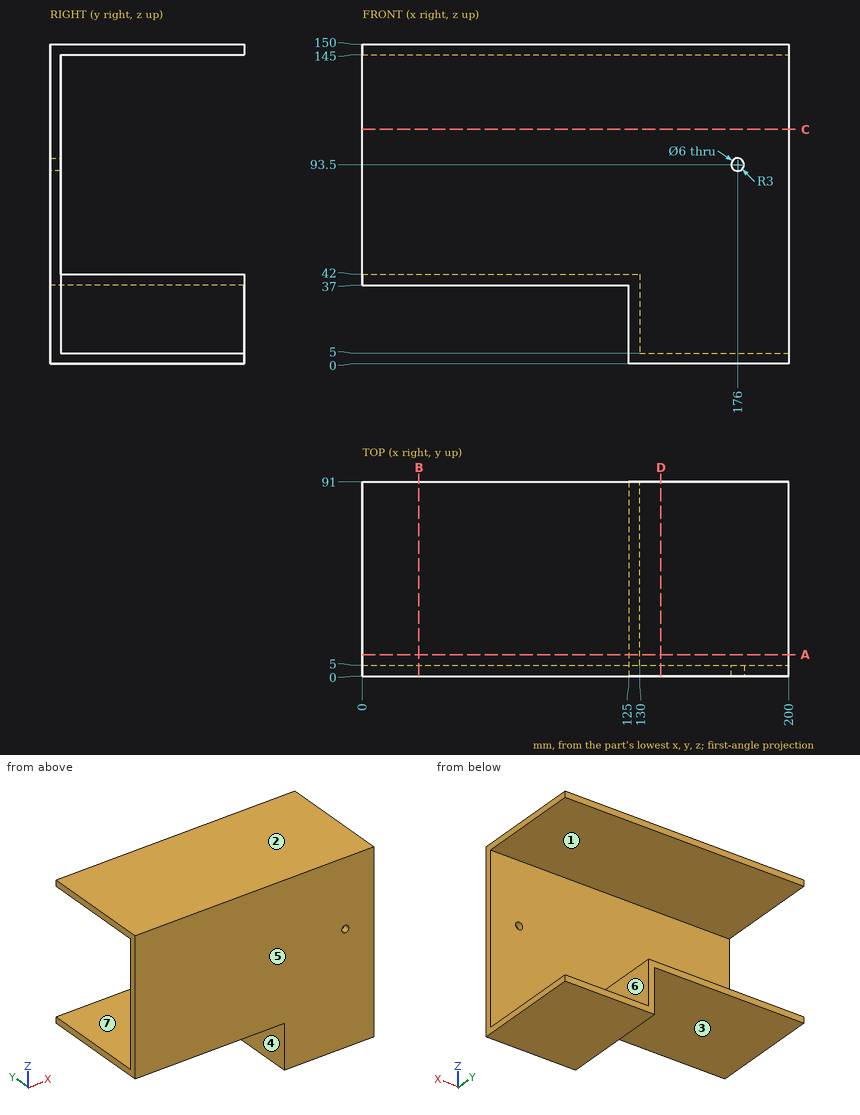
The drawing under review shows one solid part. Ordinate dimensions are in mm from its lowest x, y, z. A direction names the side the tool comes from. Round coordinates to 2 decimals unless told otherwise and drop trailing zeros. Loops run counter-clockwise (first coordinate to the right, second up) from the corner with the lowest first, then second, coordinate; pieces in that order, holes last. Notation, with made-up numbers: (9.5, -12.5) - (39.5, -12.5) arc R21 ccw to (39.5, 6.5) - close; hole circle Ø11 at (63, 5.5). An arc over 180 degrees is marked (long way). Use a Markdown table: item, result. Add a question column.
Q1. Add section B-B (x = 26.5). State the section outline as (y, z) points.
Q2. Add section D-D (x = 140). State the section outline as (y, z) points.
Q3. The part is to be moulded in two halves that separate along Z. For the marked faces 1, 2, 3 and 4, say which applies: pulls with the +Z half, pulls with the -Z half, needs draft (parallel to the pull), parting line crosses it, or undercut.
Q4. Add section C-C (z = 110). State the section outline as (x, y) points, plus the area to 3 significant figures.
Q5. Insertion check: pin 1 Ø10 at (x, y) = (128.5, 13.5) entering from -Z; pin 2 Ø10 at (x, z) = (143, 119.5) entering from +Y. Each pin has a flat end and moves straight along its axis. Give the tip position at first contact, or say it passes through.
Q6. Add section A-A (y = 10). State the section outline as (x, z) points.
Q7. Machinability: for the marked faces 5, 6 and 7, which of the approach directions +Z, -Z, +X, -X, +Y, -Y give a long, thin tool a straight path to every point of the face, cutting with its end or side? Answer none if there is none.
Q8. For probe 1 along Z at (x, y) = (96, 52); probe 2 along X at (y, z) = (2.25, 93.5); probe 3 along Z at (x, y) = (176, 3), list the stretches that pass through material, from the lowest coordinate up.
Worked answers:
| question | item | result |
|---|---|---|
| 1 | outline | (0, 37) - (91, 37) - (91, 42) - (5, 42) - (5, 145) - (91, 145) - (91, 150) - (0, 150) - close |
| 2 | outline | (0, 0) - (91, 0) - (91, 5) - (5, 5) - (5, 145) - (91, 145) - (91, 150) - (0, 150) - close |
| 3 | face 1 | undercut |
| 3 | face 2 | pulls with the +Z half |
| 3 | face 3 | pulls with the -Z half |
| 3 | face 4 | needs draft |
| 4 | outline | (0, 0) - (200, 0) - (200, 5) - (0, 5) - close |
| 4 | area | 1,000 mm² |
| 5 | pin 1 | z = 0 |
| 5 | pin 2 | y = 5 |
| 6 | outline | (0, 37) - (125, 37) - (125, 0) - (200, 0) - (200, 5) - (130, 5) - (130, 42) - (0, 42) - close; (0, 145) - (200, 145) - (200, 150) - (0, 150) - close |
| 7 | face 5 | +Z, -Z, +X, -X, -Y |
| 7 | face 6 | +X, +Y |
| 7 | face 7 | +X, -X, +Y |
| 8 | probe 1 | 37 to 42, 145 to 150 |
| 8 | probe 2 | 0 to 173, 179 to 200 |
| 8 | probe 3 | 0 to 90.5, 96.5 to 150 |
